Work out the finished part from the listing and answer in its coordinate system (mm). A direction names the side the tool comes from. Give positions to 0.01 mm unless a question says otherwise; leave off trailing zeros. Order: outer loops, then holes, each group sorted by start corner. A loop starts at its lowest first (then second) coordinate and runs counter-clockwise, first axis right, second up. Notation, with made-up numbers: (-28.75, 62.5) - (-16.75, 62.5) arc R21 cw to (-16.75, 101.5) - close; hole circle Ø10 at (10, -5.75). An arc over 180 degrees is marked (long way). Return JSON: item names as keys, results as strings. Group by question number.
from build123d import *

# Parameters (mm, degrees)
F1_DEPTH = 33.24098
F2_W     = 32.58058
F2_H     = 2.716841


with BuildPart() as f1:
    # F0 (on Front) → F1 (new body)
    with BuildSketch(Plane.XZ):
        with BuildLine():
            ThreePointArc((5.46354, 1.68862), (3.856251, 1.234842), (2.73177, 0))
            Line((2.73177, 0), (5.46354, 0))
            Line((5.46354, 0), (5.46354, 1.68862))
        make_face()
        with BuildLine():
            ThreePointArc((5.46354, 3.377241), (2.324843, 2.346928), (0, 0))
            Line((0, 0), (2.73177, 0))
            ThreePointArc((2.73177, 0), (3.856251, 1.234842), (5.46354, 1.68862))
            Line((5.46354, 1.68862), (5.46354, 3.377241))
        make_face()
    extrude(amount=-F1_DEPTH)

    # F4: sweep along a path in F3
    with BuildLine(Plane.XZ) as f4_path:
        ThreePointArc((5.46354, 1.68862), (3.506738, 1.368407), (2.071792, 0))
    # F2 (on face) → F4 (sweep, cut)
    with BuildSketch(Plane.YZ.offset(5.46354)):
        with Locations((16.62049, 1.68862)):
            Rectangle(F2_W, F2_H)
    sweep(path=f4_path.line, mode=Mode.SUBTRACT)


solid = f1.part
1. Determine the mould class of faces 3 (the flat face through (3, 0, 1)), 4 (the cylindrical face through (4.617, 16.849, 0.346)), 5 (the cylindrical face through (1.189, 16.388, 1.474)) for opening direction X: released by +X, released by -X, zero draft, split by the parting line, or undercut.
2. Consider probe 1 along Y at (x, z) = (2.9, 1.1); probe 2 along Z at (x, y) = (1.1, 29); probe 3 along Z at (x, y) = (1.15, 6.5). Determine where each line is inside the solid, lowest interval first. Write a range as from..to.
3. The part is cut by section B-B (y = 3.5). Give the vertices of the cut face in (x, z), and give its area (3 significant figures).
4. The part is cut by section C-C (z = 2.75). Give the vertices of the cut face in (x, y).
5. The part is cut by section A-A (x = 1.1). Give the vertices of the cut face in (y, z), and give its area (3 significant figures).
6. A tool of negligible diameter and unlimited length cuts with its end or side. For faces 1 (the flat face through (5.464, 16.5, 3.2)), 2 (the flat face through (1.43, 16.85, 0.25)), from which of +Z, -Z, +X, -X, +Y, -Y can it reach the whole face along a straight path? Write none if from no direction.
Answers:
{
 "1": {"face 3": "zero draft", "face 4": "undercut", "face 5": "released by -X"},
 "2": {"probe 1": "y = 0..0.33, 32.91..33.24", "probe 2": "z = 0..0.38, 0.99..1.39", "probe 3": "z = 0..0.36, 1.07..1.44"},
 "3": {"outline": "(0, 0) - (2.07, 0) - (0.81, 0.49) arc R4.71 cw to (5.46, 3.05) - (5.46, 3.38) arc R7.05 ccw to start; (3.82, 0) - (5.46, 0) - (5.46, 0.33) arc R2.02 ccw to start", "area": "2.16 mm^2"},
 "4": {"outline": "(3.07, 0) - (5.46, 0) - (5.46, 0.33) - (3.3, 0.33) - (3.3, 32.91) - (5.46, 32.91) - (5.46, 33.24) - (3.07, 33.24) - close"},
 "5": {"outline": "(0, 0) - (33.24, 0) - (33.24, 1.39) - (0, 1.39) - close; hole (0.33, 0.38) - (32.91, 0.38) - (32.91, 0.99) - (0.33, 0.99) - close", "area": "26.1 mm^2"},
 "6": {"face 1": "+Z, -Z, +X, +Y, -Y", "face 2": "none"}
}
